Geometry: final body of the model. Coordinates: model frame, mm. Face numbers are marked on the shaded views. A direction names the side the tool comes from. Give positions to 0.01 mm unless a question says otherwise; leave off trailing zeros. Write each loop counter-clockwise with the first axis right and the second up, starting at its lowest first coordinate (ties: lowest second). Pieces come first, ordered by that corner, then holes. Notation, with made-up numbers: (25.5, 52.5) - (76.5, 52.5) arc R33 cw to (76.5, 81.5) - close; hole circle Ø5 at (11, 48.5). An arc over 180 degrees is marked (long way). Return JSON: item names as keys, results as strings.
Autodesk Inventor part; units mm, degrees
ref_plane "YZ Plane" through (0, 0, 0) normal (1, 0, 0) x (0, 1, 0)
ref_plane "XZ Plane" through (0, 0, 0) normal (0, 1, 0) x (-1, 0, 0)
ref_plane "XY Plane" through (0, 0, 0) normal (0, 0, 1) x (1, 0, 0)
sketch "Sketch1" plane through (0, 0, 0) normal (0, 0, 1) x (1, 0, 0)
  line L0 (3.175, 0.8507) -> (3.175, -0.8507)
  line L1 (3.175, -0.8507) -> (2.3243, -2.3243)
  line L2 (2.3243, -2.3243) -> (0.8507, -3.175)
  line L3 (0.8507, -3.175) -> (-0.8507, -3.175)
  line L4 (-0.8507, -3.175) -> (-2.3243, -2.3243)
  line L5 (-2.3243, -2.3243) -> (-3.175, -0.8507)
  line L6 (-3.175, -0.8507) -> (-3.175, 0.8507)
  line L7 (-3.175, 0.8507) -> (-2.3243, 2.3243)
  line L8 (-2.3243, 2.3243) -> (-0.8507, 3.175)
  line L9 (-0.8507, 3.175) -> (0.8507, 3.175)
  line L10 (0.8507, 3.175) -> (2.3243, 2.3243)
  line L11 (2.3243, 2.3243) -> (3.175, 0.8507)
  line L12 (0, 0) -> (0, 3.175) construction
  dimension "d9" = 6.35
extrude "Extrusion1" add sketch "Sketch1" along normal blind 25.4 and the other way blind 25.4
sketch "Sketch2" plane through (0, 0, 0) normal (0, 1, 0) x (-1, 0, 0)
  circle A0 centre (0, 0) radius 2.286
  dimension "diamCamSlot" = 4.572
extrude "Extrusion2" add sketch "Sketch2" along normal blind 12.7
fillet "Fillet1" radius 1.5875 1 edges at (2.286, 12.7, 0)
equation "\"d9\" = camDiam"
equation "\"camDiam\" = 6.35"
properties part number "vexCamPost10"
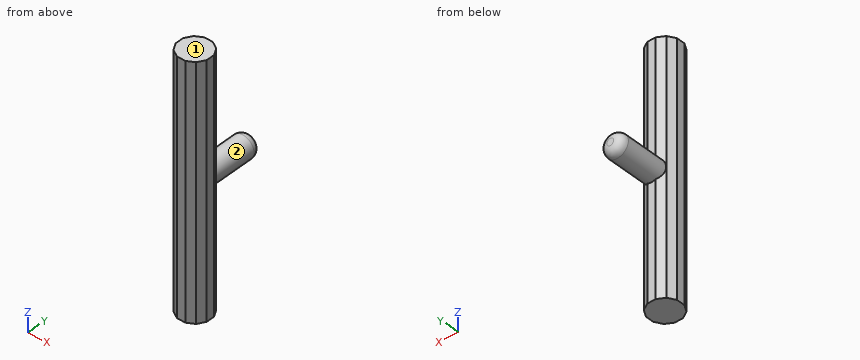
Q1. Section query A-A, the plane z = -13.5. Return the cut outline in (x, y) (3 decimals), plus the area to 3 significant figures.
Answer key:
{"outline": "(-3.175, -0.851) - (-2.324, -2.324) - (-0.851, -3.175) - (0.851, -3.175) - (2.324, -2.324) - (3.175, -0.851) - (3.175, 0.851) - (2.324, 2.324) - (0.851, 3.175) - (-0.851, 3.175) - (-2.324, 2.324) - (-3.175, 0.851) - close", "area": "32.4 mm^2"}
Q2. Material intervals for probe 1 along Z at (x, y) = (0, 11); probe 2 along Y at (x, z) = (-0.75, -17) (3 decimals); probe 3 along X at (y, z) = (1, 10), sorted ascending. Write a range as [from, to].
Answer key:
{"probe 1": "z = [-2.29, 2.29]", "probe 2": "y = [-3.175, 3.175]", "probe 3": "x = [-3.09, 3.09]"}
Q3. Section query B-B, the plane y = 7.25. Return the cut outline in (x, z).
Answer key:
{"outline": "circle Ø4.57 at (0, 0)"}
Q4. Section query C-C, the plane y = 1.75. Return the cut outline in (x, z).
Answer key:
{"outline": "(-2.66, -25.4) - (2.66, -25.4) - (2.66, 25.4) - (-2.66, 25.4) - close"}
Q5. Set-up query: the marked faces 1 and 2. Return all of +Z, -Z, +X, -X, +Y, -Y with unobstructed straight access to the full face (end or side cutting, diameter ignored); none if empty.
Answer key:
{"face 1": "+Z, +X, -X, +Y, -Y", "face 2": "+Y"}
Q6. Pin query (flat end, axial travel): P1, Ø4, axis at y = 9.5, z = -1.5, coming from the +X side; P2, Ø0.9, axis at x = 0.5, z = -16.5, coming from the +Y side (3 decimals); P3, Ø3, axis at x = 2, y = 5, coming from the -Z side; P4, Ø3, axis at x = -1, z = -15, coming from the -Y side (3 decimals). Return the tip coordinate at first contact, or that it passes through.
Answer key:
{"P1": "stops at x = 2.29", "P2": "stops at y = 3.175", "P3": "stops at z = -2.23", "P4": "stops at y = -3.175"}
